Here's how the part is built. I have some questions about the finished solid (model axes, mm). Face numbers are marked on the shaded views. A direction names the side the tool comes from. Round coordinates to 2 decimals unless told otherwise and drop trailing zeros. Loops run counter-clockwise (first coordinate to the right, second up) from the corner with the lowest first, then second, coordinate; pieces in that order, holes last. Notation, with made-up numbers: M 6,-30 L 10,-30 A7 ccw 10,-20 Z; hole C 23,-16.75 d10. An arc over 180 degrees is marked long. Answer as CSV lines item,"result".
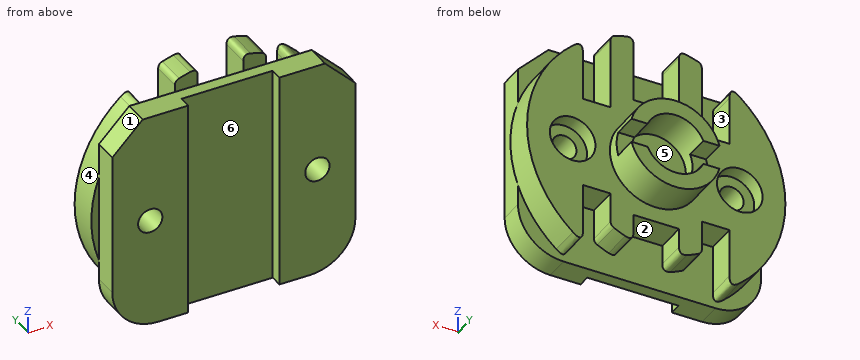
```python
from build123d import *

# Parameters (mm, degrees)
SKETCH2_W                                = 80
SKETCH2_H                                = 72
BOSS_EXTRUDE1_DEPTH                      = 8
BOSS_EXTRUDE2_DEPTH                      = 10
CHAMFER1_SIZE                            = 10
FILLET1_R                                = 15
SKETCH4_R                                = 15
SKETCH4_R_2                              = 10
BOSS_EXTRUDE3_DEPTH                      = 12
SKETCH5_W                                = 8
SKETCH5_H                                = 8
CUT_EXTRUDE1_DEPTH                       = 114.535236821
CBORE_FOR_M10_HEX_HEAD_BOLT1_D           = 8
CBORE_FOR_M10_HEX_HEAD_BOLT1_CBORE_D     = 15
CBORE_FOR_M10_HEX_HEAD_BOLT1_CBORE_DEPTH = 5
SKETCH8_W                                = 30
SKETCH8_H                                = 4
CUT_EXTRUDE2_DEPTH                       = 118.321038589


with BuildPart() as part:
    # Sketch2 → Boss-Extrude1 (new body)
    with BuildSketch(Plane(origin=(0, 0, 0), x_dir=(1, 0, 0), z_dir=(0, 1, 0))):
        with Locations((40, 36)):
            Rectangle(SKETCH2_W, SKETCH2_H)
    extrude(amount=BOSS_EXTRUDE1_DEPTH)

    # Sketch3 → Boss-Extrude2 (add)
    with BuildSketch(Plane(origin=(0, 8, 0), x_dir=(1, 0, 0), z_dir=(0, 1, 0))):
        with BuildLine():
            Line((32.5, 65.047375097), (32.5, 56))
            Line((32.5, 56), (47.5, 56))
            Line((47.5, 56), (47.5, 65.047375097))
            ThreePointArc((47.5, 65.047375097), (51.354009371, 63.768443802), (55, 61.980762114))
            Line((55, 61.980762114), (55, 51))
            Line((55, 51), (64.109126902, 51))
            Line((64.109126902, 51), (64.109126902, 71))
            ThreePointArc((64.109126902, 71), (82.5, 36), (64.109126902, 1))
            Line((64.109126902, 1), (64.109126902, 21))
            Line((64.109126902, 21), (55, 21))
            Line((55, 21), (55, -3.764934301))
            ThreePointArc((55, -3.764934301), (51.297421179, -4.970944274), (47.5, -5.833001327))
            Line((47.5, -5.833001327), (47.5, 16))
            Line((47.5, 16), (32.5, 16))
            Line((32.5, 16), (32.5, -5.833001327))
            ThreePointArc((32.5, -5.833001327), (28.702578821, -4.970944274), (25, -3.764934301))
            Line((25, -3.764934301), (25, 21))
            Line((25, 21), (15.890873098, 21))
            Line((15.890873098, 21), (15.890873098, 1))
            ThreePointArc((15.890873098, 1), (-2.5, 36), (15.890873098, 71))
            Line((15.890873098, 71), (15.890873098, 51))
            Line((15.890873098, 51), (25, 51))
            Line((25, 51), (25, 61.980762114))
            ThreePointArc((25, 61.980762114), (28.645990629, 63.768443802), (32.5, 65.047375097))
        make_face()
    extrude(amount=BOSS_EXTRUDE2_DEPTH)

    # Chamfer1
    chamfer1_edges = [part.edges().sort_by_distance(p)[0] for p in [
        (80, 4, 0),
        (0, 4, 0),
    ]]
    chamfer(chamfer1_edges, length=CHAMFER1_SIZE)

    # Fillet1
    fillet1_edges = [part.edges().sort_by_distance(p)[0] for p in [
        (0, 4, -72),
        (80, 4, -72),
    ]]
    fillet(fillet1_edges, radius=FILLET1_R)

    # Sketch4 → Boss-Extrude3 (add)
    with BuildSketch(Plane(origin=(0, 18, 0), x_dir=(1, 0, 0), z_dir=(0, 1, 0))):
        with Locations(Location((40.253775516, 36, 0), (0, 0, 270))):
            Circle(SKETCH4_R)
        with Locations(Location((40.253775516, 36, 0), (0, 0, 270))):
            Circle(SKETCH4_R_2, mode=Mode.SUBTRACT)
    extrude(amount=BOSS_EXTRUDE3_DEPTH)

    # Sketch5 → Cut-Extrude1 (cut, through all)
    with BuildSketch(Plane(origin=(0, 0, 0), x_dir=(0, 0, -1), z_dir=(1, 0, 0))):
        with Locations((36, 26)):
            Rectangle(SKETCH5_W, SKETCH5_H)
    extrude(amount=CUT_EXTRUDE1_DEPTH, mode=Mode.SUBTRACT)

    # CBORE for M10 Hex Head Bolt1 (through all)
    with Locations(Plane(origin=(0, 18, 0), x_dir=(1, 0, 0), z_dir=(0, 1, 0))):
        with Locations((67.5, 36), (12.5, 36)):
            CounterBoreHole(CBORE_FOR_M10_HEX_HEAD_BOLT1_D / 2, CBORE_FOR_M10_HEX_HEAD_BOLT1_CBORE_D / 2, CBORE_FOR_M10_HEX_HEAD_BOLT1_CBORE_DEPTH)

    # Sketch8 → Cut-Extrude2 (cut, through all)
    with BuildSketch(Plane(origin=(0, 0, -72), x_dir=(-1, 0, 0), z_dir=(0, 0, -1))):
        with Locations((-40, 2)):
            Rectangle(SKETCH8_W, SKETCH8_H)
    extrude(amount=-CUT_EXTRUDE2_DEPTH, mode=Mode.SUBTRACT)

    # Fillet2
    # a fillet whose section is not a circle: 2 mm, written as the material it takes off along each edge
    with BuildSketch(Plane(origin=(64.109126902, 8, -71), x_dir=(0.7949377645481589, 0, 0.6066909843529702), z_dir=(0, 1, 0)), Plane(origin=(15.890873098, 8, -1), x_dir=(-0.7949377645481593, 0, -0.6066909843529693), z_dir=(0, 1, 0))) as fillet2_piece_1:
        with BuildLine():
            Bezier((4.137858015, 0), (-0.159861677, 0.20946427), (2.45062112, -3.211010754), weights=[1, 1, 1])
            Line((2.45062112, -3.211010754), (0, 0))
            ThreePointArc((0, 0), (2.068929007, 0.050388308), (4.137858015, 0))
        make_face()
    extrude(amount=20.344645036, mode=Mode.SUBTRACT)
    with BuildSketch(Plane(origin=(15.890873098, 8, -71), x_dir=(-0.794937764548161, 0, 0.6066909843529674), z_dir=(0, 1, 0)), Plane(origin=(64.109126902, 8, -1), x_dir=(0.7949377645481593, 0, -0.6066909843529698), z_dir=(0, 1, 0))) as fillet2_piece_2:
        with BuildLine():
            Bezier((4.137858015, 0), (-0.159861677, -0.20946427), (2.45062112, 3.211010754), weights=[1, 1, 1])
            Line((2.45062112, 3.211010754), (0, 0))
            ThreePointArc((0, 0), (2.068929007, -0.050388308), (4.137858015, 0))
        make_face()
    extrude(amount=20.344645036, mode=Mode.SUBTRACT)
    with BuildSketch(Plane(origin=(55, 4.393986535, 3.764934301), x_dir=(0, 0, -1), z_dir=(0, 1, 0))) as fillet2_piece_3:
        with BuildLine():
            Bezier((1.408057473, 0), (-0.025844464, 0), (-0.486109283, 1.358024691), weights=[1, 1, 1])
            ThreePointArc((-0.486109283, 1.358024691), (-0.248816298, 0.676949942), (0, 0))
            Line((0, 0), (1.408057473, 0))
        make_face()
    extrude(amount=17.21202693, mode=Mode.SUBTRACT)
    with BuildSketch(Plane(origin=(47.5, 1.692392429, 5.833001327), x_dir=(0, 0, -1), z_dir=(0, 1, 0))) as fillet2_piece_4:
        with BuildLine():
            Bezier((2.462961957, 0), (-0.077040583, 0), (0.518762482, -2.469135802), weights=[1, 1, 1])
            ThreePointArc((0.518762482, -2.469135802), (0.241054451, -1.238418338), (0, 0))
            Line((0, 0), (2.462961957, 0))
        make_face()
    extrude(amount=22.615215142, mode=Mode.SUBTRACT)
    with BuildSketch(Plane(origin=(32.5, 1.692392429, 5.833001327), x_dir=(0, 0, -1), z_dir=(0, 1, 0))) as fillet2_piece_5:
        with BuildLine():
            Bezier((2.462961957, 0), (-0.077040583, 0), (0.518762482, 2.469135802), weights=[1, 1, 1])
            ThreePointArc((0.518762482, 2.469135802), (0.241054451, 1.238418338), (0, 0))
            Line((0, 0), (2.462961957, 0))
        make_face()
    extrude(amount=22.615215142, mode=Mode.SUBTRACT)
    with BuildSketch(Plane(origin=(25, 4.393986535, 3.764934301), x_dir=(0, 0, -1), z_dir=(0, 1, 0))) as fillet2_piece_6:
        with BuildLine():
            Bezier((1.408057473, 0), (-0.025844464, 0), (-0.486109283, -1.358024691), weights=[1, 1, 1])
            ThreePointArc((-0.486109283, -1.358024691), (-0.248816298, -0.676949942), (0, 0))
            Line((0, 0), (1.408057473, 0))
        make_face()
    extrude(amount=17.21202693, mode=Mode.SUBTRACT)
    with BuildSketch(Plane(origin=(55, 8, -61.980762114), x_dir=(0, 0, 1), z_dir=(0, 1, 0))) as fillet2_piece_7:
        with BuildLine():
            Bezier((1.181568578, 0), (-0.02814818, 0), (-0.589802389, -1.071428571), weights=[1, 1, 1])
            ThreePointArc((-0.589802389, -1.071428571), (-0.30036176, -0.532708341), (0, 0))
            Line((0, 0), (1.181568578, 0))
        make_face()
    extrude(amount=13.057599182, mode=Mode.SUBTRACT)
    with BuildSketch(Plane(origin=(47.5, 8, -65.047375097), x_dir=(0, 0, 1), z_dir=(0, 1, 0))) as fillet2_piece_8:
        with BuildLine():
            Bezier((2.708240714, 0), (-0.139233273, 0), (0.826873973, 2.678571429), weights=[1, 1, 1])
            ThreePointArc((0.826873973, 2.678571429), (0.382133114, 1.348949208), (0, 0))
            Line((0, 0), (2.708240714, 0))
        make_face()
    extrude(amount=17.008238663, mode=Mode.SUBTRACT)
    with BuildSketch(Plane(origin=(32.5, 8, -65.047375097), x_dir=(-0.9555080660857783, 0, 0.294964973590113), z_dir=(0, 1, 0))) as fillet2_piece_9:
        with BuildLine():
            Bezier((2.803295465, 0), (-0.041068939, -0.133038515), (0.798836151, 2.587745848), weights=[1, 1, 1])
            Line((0.798836151, 2.587745848), (0, 0))
            ThreePointArc((0, 0), (1.401647733, -0.032761495), (2.803295465, 0))
        make_face()
    extrude(amount=17.008238663, mode=Mode.SUBTRACT)
    with BuildSketch(Plane(origin=(25, 8, -61.980762114), x_dir=(0, 0, 1), z_dir=(0, 1, 0))) as fillet2_piece_10:
        with BuildLine():
            Bezier((1.181568578, 0), (-0.02814818, 0), (-0.589802389, 1.071428571), weights=[1, 1, 1])
            ThreePointArc((-0.589802389, 1.071428571), (-0.30036176, 0.532708341), (0, 0))
            Line((0, 0), (1.181568578, 0))
        make_face()
    extrude(amount=13.057599182, mode=Mode.SUBTRACT)


solid = part.part
```
1. I want a section at C-C, the plane z = -54.5. Please give me the cut outline in (x, y).
Evaluation:
outline,"M 0,0 L 25,0 L 25,4 L 55,4 L 55,0 L 80,0 L 80,8 L 78.26,8 L 78.26,18 L 64.11,18 L 64.11,8 L 55,8 L 55,18 L 25,18 L 25,8 L 15.89,8 L 15.89,18 L 1.74,18 L 1.74,8 L 0,8 Z"
2. I want a section at B-B, the plane z = -17. Please give me the cut outline in (x, y), and give its area (3 significant figures).
Evaluation:
outline,"M 0,0 L 25,0 L 25,4 L 55,4 L 55,0 L 80,0 L 80,8 L 78.02,8 L 78.02,18 L 64.11,18 L 64.11,8 L 55,8 L 55,18 L 25,18 L 25,8 L 15.89,8 L 15.89,18 L 1.98,18 L 1.98,8 L 0,8 Z"
area,"1,100 mm²"
3. For P1, Ø3, axis at y = 11.5, z = -10.5, coming from the +X side; P2, Ø4, axis at x = 29, z = -62.5, coming from the +Y side; P3, Ø2, axis at y = 1.5, z = -33.5, coming from the +X side, each with a flat end and sliding along its axis, tell me the tip position at first contact or that it passes through.
Evaluation:
P1,"stops at x = 75.07"
P2,"stops at y = 18"
P3,"stops at x = 80"
4. If I drill on line 1 (X direction, y = 16.2, z = -36); line 2 (X direction, y = 4.25, z = -36); line 3 (Z direction, x = 44, y = 9.25), over which ranges is the centre line in solid material (lowest first)? Write a range as [from, to].
Evaluation:
line 1,"x = [-2.5, 5], [20, 60], [75, 82.5]"
line 2,"x = [0, 8.5], [16.5, 63.5], [71.5, 80]"
line 3,"z = [-56, -16]"
5. We'd pull the mould along Z, two halves only. Please class the marked faces 4, 5 and 6: pulls with the +Z half, pulls with the -Z half, needs draft (parallel to the pull), parting line crosses it, or undercut.
Evaluation:
face 4,"parting line crosses it"
face 5,"undercut"
face 6,"needs draft"
6. Which directions (+Z, -Z, +X, -X, +Y, -Y) give clear straight access to the entire face, cutting with the end or side of a thin tool? Please do the marked faces 1, 2 and 3.
Evaluation:
face 1,"+Z, -X, +Y, -Y"
face 2,"-Z, +Y"
face 3,"+Z, +Y"
7. I want a section at A-A, the plane z = -36. Count the separate pieces of the cut face and the enclosed holes in it, and give its area (3 significant figures).
Evaluation:
separate pieces,"3"
enclosed holes,"0"
area,"1,050 mm²"
